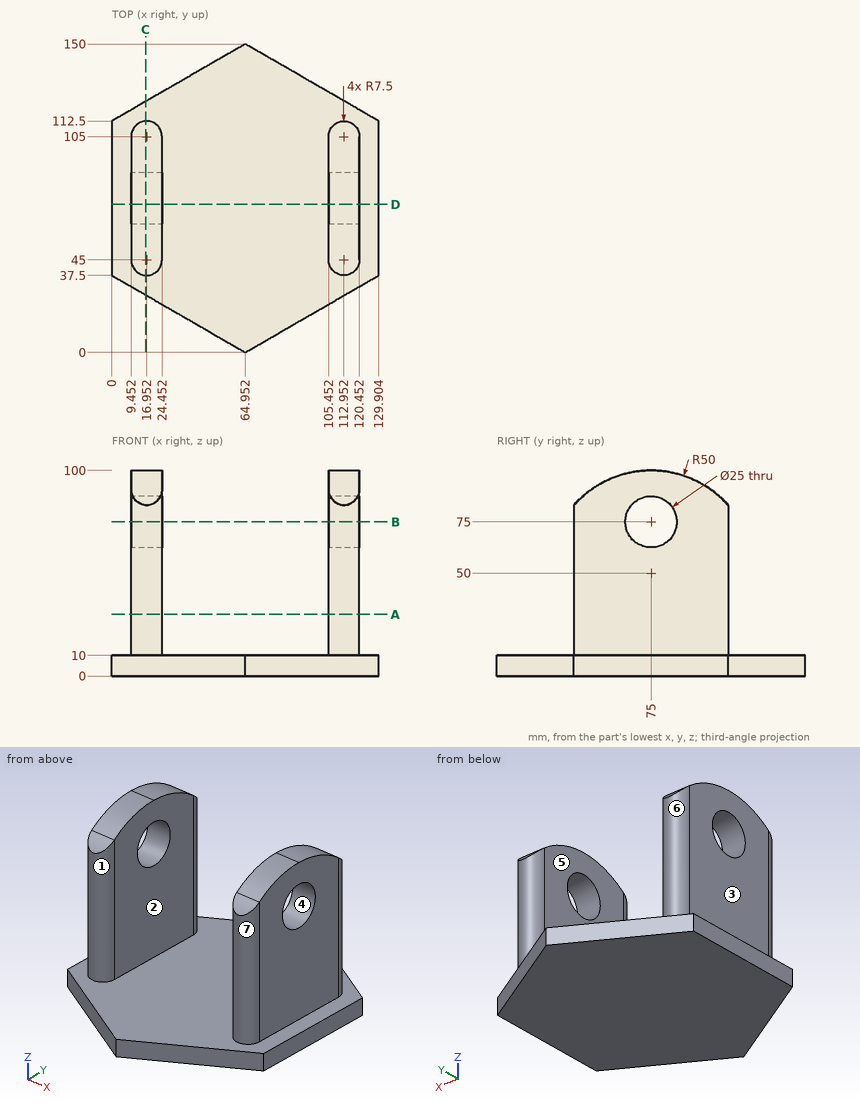
Input: dimensioned drawing with shaded views. Units: mm. Origin: part minimum x, y, z. A direction names the side the tool comes from. Give positions to 0.01 mm unless a question says otherwise; leave off trailing zeros. Order: outer loops, then holes, each group sorted by start corner. A loop starts at its lowest first (then second) coordinate and runs counter-clockwise, first axis right, second up.
(1) Access query for the marked faces 5, 6 and 7. Directions: +Z, -Z, +X, -X, +Y, -Y. A direction counts if a zero-diameter tool reaches every point of the face in a straight line with its end or side. Return the directions, or none.
(2) Section query D-D (y = 72). Return the cut outline in (x, z) (1 decimal), plus the area to 3 significant figures.
(3) Section query A-A (z = 30). Return the cut outline in (x, y).
(4) Section query C-C (x = 16.5). Return the cut outline in (y, z).
(5) Contact query for flat-ended pins moving along their axis: P1, Ø10, axis at x = 26, y = 26, coming from the +Z side; P2, Ø5, axis at x = 70, z = 12, coming from the -Y side; P3, Ø4, axis at x = 104.5, y = 105, coming from the +Z side. Output: stop coordinate, or through.
(6) Material intervals for line 1 along Z through (x, y) = (113, 75); line 2 along X through (y, z) = (74, 38); line 3 along Z through (x, y) = (27.5, 114), sorted ascending.
(7) Pull-direction query (X, two-part tool) for the marked faces 1, 2, 3 and 4; classes: +X half, -X half, draft (parallel to the pull), parting line (faces both ways), or undercut.
(8) Section query B-B (z = 75). Return the cut outline in (x, y).
Outcome:
1. face 5: +Z, +Y, -Y
1. face 6: +Z, +Y
1. face 7: +Z, -Y
2. outline: (0, 0) - (129.9, 0) - (129.9, 10) - (120.5, 10) - (120.5, 62.9) - (105.5, 62.9) - (105.5, 10) - (24.5, 10) - (24.5, 62.9) - (9.5, 62.9) - (9.5, 10) - (0, 10) - close; (9.5, 87.1) - (24.5, 87.1) - (24.5, 99.9) - (9.5, 99.9) - close; (105.5, 87.1) - (120.5, 87.1) - (120.5, 99.9) - (105.5, 99.9) - close
2. area: 3,270 mm2
3. outline: (9.45, 45) arc R7.5 ccw to (24.45, 45) - (24.45, 105) arc R7.5 ccw to (9.45, 105) - close; (105.45, 45) arc R7.5 ccw to (120.45, 45) - (120.45, 105) arc R7.5 ccw to (105.45, 105) - close
4. outline: (27.97, 0) - (122.03, 0) - (122.03, 10) - (112.49, 10) - (112.49, 83.09) arc R50 ccw to (37.51, 83.09) - (37.51, 10) - (27.97, 10) - close; hole circle Ø25 at (75, 75)
5. P1: stops at z = 10
5. P2: stops at y = 2.05
5. P3: stops at z = 91.26
6. line 1: z = 0 to 62.5, 87.5 to 100
6. line 2: x = 9.45 to 24.45, 105.45 to 120.45
6. line 3: z = 0 to 10
7. face 1: undercut
7. face 2: undercut
7. face 3: -X half
7. face 4: draft
8. outline: (9.45, 45) arc R7.5 ccw to (24.45, 45) - (24.45, 62.5) - (9.45, 62.5) - close; (9.45, 87.5) - (24.45, 87.5) - (24.45, 105) arc R7.5 ccw to (9.45, 105) - close; (105.45, 45) arc R7.5 ccw to (120.45, 45) - (120.45, 62.5) - (105.45, 62.5) - close; (105.45, 87.5) - (120.45, 87.5) - (120.45, 105) arc R7.5 ccw to (105.45, 105) - close
